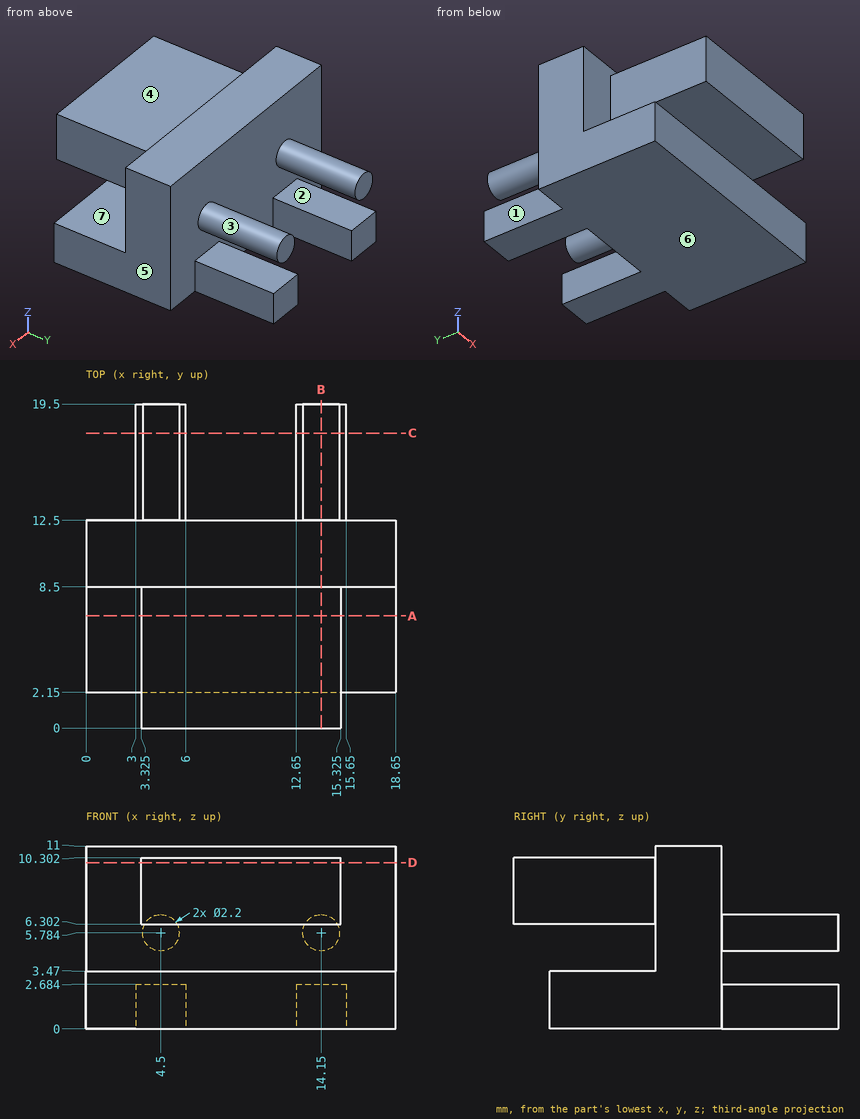
Source: three-view drawing plus pictorial views. Frame: mm from the lowest corner of the part. A direction names the side the tool comes from. Coordinates: 2 decimals unless noted, no trailing zeros. Order: outer loops, then holes, each group sorted by start corner. A loop starts at its lowest first (then second) coordinate and runs counter-clockwise, first axis right, second up.
Item 1: Cut plane B-B (x = 14.15). Return loops of the section in (y, z), plus the area to 3 significant figures.
Output values:
outline: (0, 6.3) - (8.5, 6.3) - (8.5, 3.47) - (2.15, 3.47) - (2.15, 0) - (19.5, 0) - (19.5, 2.68) - (12.5, 2.68) - (12.5, 4.68) - (19.5, 4.68) - (19.5, 6.88) - (12.5, 6.88) - (12.5, 11) - (8.5, 11) - (8.5, 10.3) - (0, 10.3) - close
area: 134 mm2
Item 2: Cut plane D-D (z = 10). Return loops of the section in (x, y) (3 decimals).
Output values:
outline: (0, 8.5) - (3.325, 8.5) - (3.325, 0) - (15.325, 0) - (15.325, 8.5) - (18.65, 8.5) - (18.65, 12.5) - (0, 12.5) - close
Item 3: Material intervals for line 1 (Z direction, x = 6, y = 5.75); line 2 (X direction, y = 13.5, z = 2.25); line 3 (Y direction, x = 6.75, z = 9), sorted ascending.
Output values:
line 1: z = 0 to 3.47, 6.3 to 10.3
line 2: x = 3 to 6, 12.65 to 15.65
line 3: y = 0 to 12.5
Item 4: First-contact query: P1, Ø4.5, axis at y = 5.5, z = 7.5, coming from the -X side (3 decimals); P2, Ø3, axis at x = 12, z = 2, coming from the -Y side; P3, Ø2, axis at y = 16, z = 0.5, coming from the +X side. Flat tips, straight axial feed; report the tip coordinate or a pass-through.
Output values:
P1: stops at x = 3.325
P2: stops at y = 2.15
P3: stops at x = 15.65
Item 5: Cut plane C-C (y = 17.75). Return loops of the section in (x, z).
Output values:
outline: (3, 0) - (6, 0) - (6, 2.68) - (3, 2.68) - close; circle Ø2.2 at (4.5, 5.78); (12.65, 0) - (15.65, 0) - (15.65, 2.68) - (12.65, 2.68) - close; circle Ø2.2 at (14.15, 5.78)
Item 6: Pull-direction query (Z, two-part tool) for the marked faces 5, 6 and 7; classes: pulls with the +Z half, pulls with the -Z half, needs draft (parallel to the pull), parting line crosses it, or undercut.
Output values:
face 5: needs draft
face 6: pulls with the -Z half
face 7: undercut
Item 7: Set-up query: the marked faces 1, 2, 3 and 4. Return all of +Z, -Z, +X, -X, +Y, -Y with unobstructed straight access to the full face (end or side cutting, diameter ignored); none if empty.
Output values:
face 1: +Z, -Z, -X, +Y
face 2: +X, -X, +Y
face 3: +Y
face 4: +Z, +X, -X, -Y
Item 8: Cut plane A-A (y = 6.75). Return loops of the section in (x, z) (3 decimals), plus the area to 3 significant figures.
Output values:
outline: (0, 0) - (18.65, 0) - (18.65, 3.47) - (0, 3.47) - close; (3.325, 6.302) - (15.325, 6.302) - (15.325, 10.302) - (3.325, 10.302) - close
area: 113 mm2
